```python
from build123d import *

# Parameters (mm, degrees)
BOSS_EXTRUDE1_DEPTH = 400
CHAMFER1_SIZE       = 0.5
LPATTERN1_COUNT     = 10
LPATTERN1_PITCH     = 40


with BuildPart() as part:
    # Sketch1 → Boss-Extrude1 (new body)
    with BuildSketch(Plane.XY):
        with BuildLine():
            Line((-7.5, 10), (7.5, 10))
            Line((7.5, 10), (7.5, 8.25))
            Line((7.5, 8.25), (7.5, 8.030776406))
            ThreePointArc((7.5, 8.030776406), (6.865647614, 7.812463569), (6.5, 7.25))
            Line((6.5, 7.25), (6, 7.25))
            Line((6, 7.25), (6, 6.75))
            Line((6, 6.75), (6.5, 6.75))
            ThreePointArc((6.5, 6.75), (6.865647614, 6.187536431), (7.5, 5.969223594))
            Line((7.5, 5.969223594), (7.5, 5.75))
            Line((7.5, 5.75), (7.5, 0))
            Line((7.5, 0), (-7.5, 0))
            Line((-7.5, 0), (-7.5, 5.75))
            Line((-7.5, 5.75), (-7.5, 5.969223594))
            ThreePointArc((-7.5, 5.969223594), (-6.865647614, 6.187536431), (-6.5, 6.75))
            Line((-6.5, 6.75), (-6, 6.75))
            Line((-6, 6.75), (-6, 7.25))
            Line((-6, 7.25), (-6.5, 7.25))
            ThreePointArc((-6.5, 7.25), (-6.865647614, 7.812463569), (-7.5, 8.030776406))
            Line((-7.5, 8.030776406), (-7.5, 8.25))
            Line((-7.5, 8.25), (-7.5, 10))
        make_face()
    extrude(amount=BOSS_EXTRUDE1_DEPTH)

    # Chamfer1
    chamfer1_edges = [part.edges().sort_by_distance(p)[0] for p in [
        (-7.5, 10, 200),
        (7.5, 10, 200),
        (7.5, 0, 200),
        (-7.5, 0, 200),
    ]]
    chamfer(chamfer1_edges, length=CHAMFER1_SIZE)

    # Sketch3 → M3 六角承窩頭蓋螺釘的柱孔1 (revolve, cut)
    with BuildSketch(Plane(origin=(0, 10, 15), x_dir=(0, 0, 1), z_dir=(1, 0, 0))):
        Polygon((0, 0), (0, 10), (2, 10), (1.75, 9.75), (1.75, 4.5), (3, 4.5), (3, 0.5), (3.5, 0), align=None)
    hole_wizard_m3_1 = revolve(axis=Axis((0, 16.35, 15), (0, -1, 0)), mode=Mode.SUBTRACT)

    # LPattern1: M3 六角承窩頭蓋螺釘的柱孔1 ×10
    with Locations(*[(0, 0, i * LPATTERN1_PITCH) for i in range(1, LPATTERN1_COUNT)]):
        add(hole_wizard_m3_1, mode=Mode.SUBTRACT)


solid = part.part
```
CAD build for the part. Positions are in the model's coordinates, mm. Coordinates: 2 decimals unless noted, no trailing zeros. Order: outer loops, then holes, each group sorted by start corner. A loop starts at its lowest first (then second) coordinate and runs counter-clockwise, first axis right, second up. Notation, with made-up numbers: (48.5, 12) -> (90.5, 12) arc R33 cw to (90.5, 49) -> close; hole circle Ø3 at (6, 56). An arc over 180 degrees is marked (long way). Use one line per item in the form item = value. Start each with the question number.
1) Band-saw the part on A-A on y = 4. State how many separate pieces and enclosed holes the cut face has, then the cut area to 3 significant figures.
2) Drop a flat-ended pin along its axis: pin 1 (1.8 mm diameter, centred on x = -0.5, z = 136.5, fed in from +Y). Give the stop position or say it passes through.
3) Band-saw the part on B-B on z = 234.5. Give the cut face in (x, y), then the cut area to 3 significant figures.
4) Drill centre lines: L1, parallel to X at y = 8.55, z = 335; L2, parallel to Y at x = 6.75, z = 184.5; L3, parallel to X at y = 7.75, z = 49.5. Where is each one in solid material? Low to high. Write a range as [from, to].
Entries:
q1.separate_pieces = 1
q1.enclosed_holes = 10
q1.area = 5,900 mm2
q2.pin_1 = 5.5
q3.outline = (-7.5, 0.5) -> (-7, 0) -> (7, 0) -> (7.5, 0.5) -> (7.5, 5.97) arc R1.03 cw to (6.5, 6.75) -> (6, 6.75) -> (6, 7.25) -> (6.5, 7.25) arc R1.03 cw to (7.5, 8.03) -> (7.5, 9.5) -> (7, 10) -> (-7, 10) -> (-7.5, 9.5) -> (-7.5, 8.03) arc R1.03 cw to (-6.5, 7.25) -> (-6, 7.25) -> (-6, 6.75) -> (-6.5, 6.75) arc R1.03 cw to (-7.5, 5.97) -> close
q3.area = 146 mm2
q4.L1 = [-7.5, -3], [3, 7.5]
q4.L2 = [0, 6.29], [7.71, 10]
q4.L3 = [-6.79, 6.79]
